```python
from build123d import *

# Parameters (mm, degrees)
CUT_EXTRUDE1_DEPTH = 52.59692143


with BuildPart() as part:
    # Sketch2 → Revolve1 (revolve)
    with BuildSketch(Plane.XY):
        with BuildLine():
            Line((-25, 0), (-25, 7.218127455))
            ThreePointArc((-25, 7.218127455), (-24.486963528, 8.469250598), (-23.243251097, 9))
            ThreePointArc((-23.243251097, 9), (-15.040879193, 8.611248064), (-6.94833646, 7.218127455))
            ThreePointArc((-6.94833646, 7.218127455), (0, 6.408356031), (6.94833646, 7.218127455))
            ThreePointArc((6.94833646, 7.218127455), (15.040879193, 8.611248064), (23.243251097, 9))
            ThreePointArc((23.243251097, 9), (24.486963528, 8.469250598), (25, 7.218127455))
            Line((25, 7.218127455), (25, 0))
            Line((25, 0), (-25, 0))
        make_face()
    revolve(axis=Axis((25, 0, 0), (-1, 0, 0)))

    # Sketch3 → Cut-Extrude1 (cut, through all)
    with BuildSketch(Plane(origin=(25, 0, 0), x_dir=(0, 0, -1), z_dir=(1, 0, 0))):
        Polygon((3.117691454, 0), (1.558845727, 2.7), (-1.558845727, 2.7), (-3.117691454, 0), (-1.558845727, -2.7), (1.558845727, -2.7), align=None)
    extrude(amount=-CUT_EXTRUDE1_DEPTH, mode=Mode.SUBTRACT)


solid = part.part
```
Check sheet for the modelled part. Datum: model origin and axes. Units: mm. A direction names the side the tool comes from. Give positions to 0.01 mm unless a question says otherwise; leave off trailing zeros. Write each loop counter-clockwise with the first axis right and the second up, starting at its lowest first coordinate (ties: lowest second). Pieces come first, ordered by that corner, then holes. Notation, with made-up numbers: (-7, 89.25) - (25, 89.25) arc R8 ccw to (25, 101.25) - close; hole circle Ø8 at (43, 16). An arc over 180 degrees is marked (long way). Answer as a JSON object with one key per item and string values. Group by question number.
1) Sectioned sample at A-A (x = -0.5). Record the cut outline in (y, z), then the cut area to 3 significant figures.
2) Depth check by flat-ended pin: P1, Ø5, axis at x = 5.5, z = -4.5, coming from the -Y side; P2, Ø2.5, axis at x = 11, z = 0.5, coming from the -Y side; P3, Ø4, axis at x = -11.5, y = -7, coming from the +Z side. Enter the tip coordinate at first touch or a pass-through.
3) Access from +Z, -Z, +X, -X, +Y, -Y to the whole of each face (thin tool, end or side, straight path). Record for faces 3 (the face through (25, 3, 0)), 4 (the face through (0.35, -1.369, -2.327)).
4) Thickness scan on probe 1 along Y at (x, z) = (19.5, 2.5); probe 2 along Z at (x, y) = (-5.5, 0.5); probe 3 along Z at (x, y) = (4.5, -0.25). Record the ranges inside material, lowest first. Write a range as from..to.
5) Release check for a two-part mould opening along Y. For faces 1 (the face through (0.35, -1.33, 2.35)), 2 (the face through (-25, -3, 0)) record: pulls with the +Y half, pulls with the -Y half, needs draft (parallel to the pull), parting line crosses it, or undercut.
Geometry results:
{
 "1": {"outline": "circle Ø12.82 at (0, 0); hole (-2.7, -1.56) - (0, -3.12) - (2.7, -1.56) - (2.7, 1.56) - (0, 3.12) - (-2.7, 1.56) - close", "area": "104 mm^2"},
 "2": {"P1": "stops at y = -6.79", "P2": "stops at y = -8.24", "P3": "stops at z = 6.46"},
 "3": {"face 3": "+Z, -Z, +X, +Y, -Y", "face 4": "+X, -X"},
 "4": {"probe 1": "y = -8.59..-1.07, 1.07..8.59", "probe 2": "z = -6.9..-2.83, 2.83..6.9", "probe 3": "z = -6.74..-2.97, 2.97..6.74"},
 "5": {"face 1": "undercut", "face 2": "needs draft"}
}
